Input: dimensioned drawing with shaded views. Units: mm. Origin: part minimum x, y, z. A direction names the side the tool comes from. Give positions to 0.01 mm unless a question says otherwise; leave off trailing zeros. Loops run counter-clockwise (first coordinate to the right, second up) from the corner with the lowest first, then second, coordinate; pieces in that order, holes last. Notation, with made-up numbers: (14, -14.75) -> (64, -14.75) arc R29 ccw to (64, 11.25) -> close; hole circle Ø1 at (88, 20). An arc over 180 degrees is marked (long way). Answer as a JSON object with one key per item and string values.
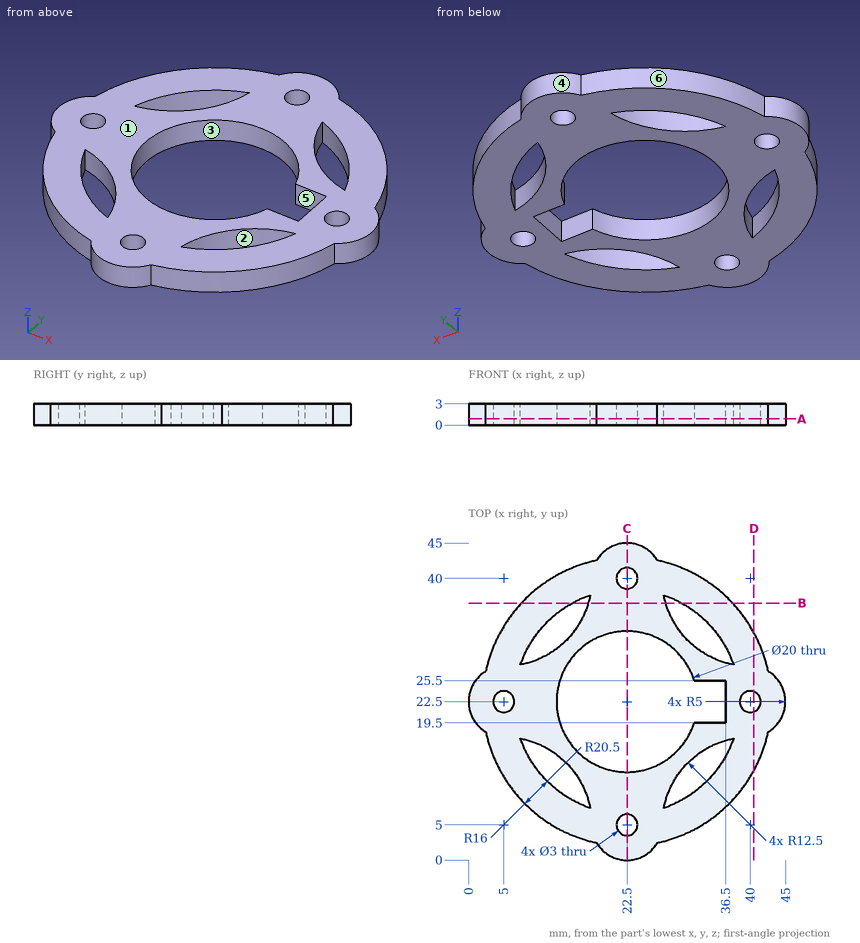
Q1. Section C-C, the plane x = 22.5. Return the cut outline in (y, z).
Evaluation:
{"outline": "(0, 0) -> (3.5, 0) -> (3.5, 3) -> (0, 3) -> close; (6.5, 0) -> (12.5, 0) -> (12.5, 3) -> (6.5, 3) -> close; (32.5, 0) -> (38.5, 0) -> (38.5, 3) -> (32.5, 3) -> close; (41.5, 0) -> (45, 0) -> (45, 3) -> (41.5, 3) -> close"}
Q2. Pin query (flat end, axial travel): pin 1 (0.9 mm diameter, centred on x = 34, z = 1.5, fed in from +Y); pin 2 (1.5 mm diameter, centred on x = 21, z = 0.5, fed in from +Y); pin 3 (1.5 mm diameter, centred on y = 19.5, z = 2, fed in from -X). Return the tip coordinate at first contact, or that it passes through.
Evaluation:
{"pin 1": "stops at y = 39.77", "pin 2": "stops at y = 44.94", "pin 3": "stops at x = 0.53"}
Q3. Section B-B, the plane y = 36.5. Return the cut outline in (x, z), then the cut area to 3 significant figures.
Evaluation:
{"outline": "(7.53, 0) -> (14.75, 0) -> (14.75, 3) -> (7.53, 3) -> close; (17, 0) -> (28, 0) -> (28, 3) -> (17, 3) -> close; (30.25, 0) -> (37.47, 0) -> (37.47, 3) -> (30.25, 3) -> close", "area": "76.4 mm2"}
Q4. Section A-A, the plane z = 0.9. Give the number of separate pieces and of enclosed holes in the cut face, then the cut area to 3 significant figures.
Evaluation:
{"separate pieces": "1", "enclosed holes": "9", "area": "860 mm2"}
Q5. Ray query, line 1 along Y through (x, z) = (22.5, 2); line 2 along X through (y, z) = (28.5, 1.1); line 3 along Y through (x, z) = (29, 1.1). Return the intervals inside material, ascending.
Evaluation:
{"line 1": "y = 0 to 3.5, 6.5 to 12.5, 32.5 to 38.5, 41.5 to 45", "line 2": "x = 2.9 to 7.67, 9.9 to 14.5, 30.5 to 35.1, 37.33 to 42.1", "line 3": "y = 3.06 to 7.88, 10.94 to 14.9, 30.1 to 34.06, 37.12 to 41.94"}
Q6. Section D-D, the plane x = 40.5. Return the cut outline in (y, z), then the cut area to 3 significant figures.
Evaluation:
{"outline": "(12.69, 0) -> (21.09, 0) -> (21.09, 3) -> (12.69, 3) -> close; (23.91, 0) -> (32.31, 0) -> (32.31, 3) -> (23.91, 3) -> close", "area": "50.4 mm2"}
Q7. Draft query along X for the marked faces 1, 2, 3 and 4. Return one class per face: +X half, -X half, draft (parallel to the pull), parting line (faces both ways), or undercut.
Evaluation:
{"face 1": "draft", "face 2": "undercut", "face 3": "undercut", "face 4": "parting line"}
Q8. Access query for the marked faces 5 and 6. Directions: +Z, -Z, +X, -X, +Y, -Y. A direction counts if a zero-diameter tool reaches every point of the face in a straight line with its end or side. Return the directions, or none.
Evaluation:
{"face 5": "+Z, -Z", "face 6": "+Z, -Z, -X, +Y"}
